Verification items for the finished model (mm, model axes). A direction names the side the tool comes from. Round coordinates to 2 decimals unless told otherwise and drop trailing zeros. Loops run counter-clockwise (first coordinate to the right, second up) from the corner with the lowest first, then second, coordinate; pieces in that order, holes last. Notation, with made-up numbers: (13.25, 2.25) -> (58.25, 2.25) arc R20 cw to (58.25, 37.25) -> close; hole circle Ø9 at (-21, 36). An arc over 180 degrees is marked (long way). Write item = value, one per line.
```python
from build123d import *

# Parameters (mm, degrees)
SKETCH_1_W      = 20
SKETCH_1_H      = 115
SKETCH_1_W_2    = 80
SKETCH_1_H_2    = 20
EXTRUDE_1_DEPTH = 55


with BuildPart() as part:
    # Эскиз1 → Бобышка-Вытянуть1 (new, symmetric)
    with BuildSketch(Plane(origin=(0, 0, 0), x_dir=(0, 0, -1), z_dir=(1, 0, 0))):
        Rectangle(SKETCH_1_W, SKETCH_1_H)
        with Locations((50, -47.5)):
            Rectangle(SKETCH_1_W_2, SKETCH_1_H_2)
        with Locations((50, 27.5)):
            Rectangle(SKETCH_1_W_2, SKETCH_1_H_2)
    extrude(amount=EXTRUDE_1_DEPTH, both=True)


solid = part.part
```
(1) Draft check along Y on faces 1 (the face through (1, -57.5, -39)), 2 (the face through (1, 57.5, 0)), 3 (the face through (55, -12, -6)), 4 (the face through (1, -10, -10)). Enter one of: released by +Y, released by -Y, zero draft, split by the parting line, or undercut.
Filled sheet:
face_1 = released by -Y
face_2 = released by +Y
face_3 = zero draft
face_4 = undercut
(2) Sectioned sample at C-C, the plane y = -30. Record the cut outline in (x, z), and give its area (3 significant figures).
Filled sheet:
outline = (-55, -10) -> (55, -10) -> (55, 10) -> (-55, 10) -> close
area = 2,200 mm2
(3) Set-up check for faces 5 (the face through (1, 47, -10)), 6 (the face through (1, -37.5, -49)), 7 (the face through (-55, -12, -6)): record each of +Z, -Z, +X, -X, +Y, -Y from which the full face is reachable in a straight line by a thin tool's end or side.
Filled sheet:
face_5 = -Z, +X, -X, +Y
face_6 = -Z, +X, -X
face_7 = +Z, -Z, -X, +Y, -Y
(4) Go/stop test with flat-tipped pins: pin 1 Ø6 at (x, y) = (-19, -9.5) entering from -Z; pin 2 Ø1 at (x, z) = (33, -51.5) entering from +Y. Record where each tip stops, or that it passes through.
Filled sheet:
pin_1 = -10
pin_2 = 37.5
(5) Material ranges on probe 1 along Y at (x, z) = (-14.5, -36); probe 2 along Z at (x, y) = (21.5, 7.5), recorded low to high. Write a range as from..to.
Filled sheet:
probe_1 = -57.5..-37.5, 17.5..37.5
probe_2 = -10..10
(6) Sectioned sample at A-A, the plane z = -29. Record the cut outline in (x, y).
Filled sheet:
outline = (-55, -57.5) -> (55, -57.5) -> (55, -37.5) -> (-55, -37.5) -> close; (-55, 17.5) -> (55, 17.5) -> (55, 37.5) -> (-55, 37.5) -> close
(7) Sectioned sample at B-B, the plane x = -41. Record the cut outline in (y, z).
Filled sheet:
outline = (-57.5, -90) -> (-37.5, -90) -> (-37.5, -10) -> (17.5, -10) -> (17.5, -90) -> (37.5, -90) -> (37.5, -10) -> (57.5, -10) -> (57.5, 10) -> (-57.5, 10) -> close
